from build123d import *

# Parameters (mm, degrees)
SKETCH1_R           = 6.7945
BOSS_EXTRUDE1_DEPTH = 25.4
SKETCH2_W           = 13.589
SKETCH2_H           = 1.500538131
BOSS_EXTRUDE2_DEPTH = 13.97
BOSS_EXTRUDE3_DEPTH = 25.4
CUT_EXTRUDE1_DEPTH  = 27.94


with BuildPart() as part:
    # Sketch1 → Boss-Extrude1 (new body)
    with BuildSketch(Plane.XY):
        Circle(SKETCH1_R)
    extrude(amount=-BOSS_EXTRUDE1_DEPTH)

    # Sketch2 → Boss-Extrude2 (add)
    with BuildSketch(Plane(origin=(0, 0, 0), x_dir=(1, 0, 0), z_dir=(0, 1, 0))):
        with Locations((0, 24.649730935)):
            Rectangle(SKETCH2_W, SKETCH2_H)
    extrude(amount=BOSS_EXTRUDE2_DEPTH)

    # Sketch6 → Boss-Extrude3 (add)
    with BuildSketch(Plane(origin=(0, 13.97, 0), x_dir=(1, 0, 0), z_dir=(0, 1, 0))):
        Polygon((-20.876229987, 25.399999851), (18.493770013, 25.40000027), (18.6055, 0), (-20.876229987, 0), align=None)
    extrude(amount=BOSS_EXTRUDE3_DEPTH)

    # Sketch11 → Cut-Extrude1 (cut)
    with BuildSketch(Plane.XY):
        Polygon((0, 21.022742384), (-12.580876385, 21.022742384), (-12.580876385, 29.426569926), (-6.246648163, 29.426569926), (-6.246648163, 39.37), (0, 39.37), (6.233662889, 39.37), (6.233662889, 29.426569926), (12.693321373, 29.426569926), (12.693321373, 21.022742384), align=None)
    extrude(amount=-CUT_EXTRUDE1_DEPTH, mode=Mode.SUBTRACT)


solid = part.part
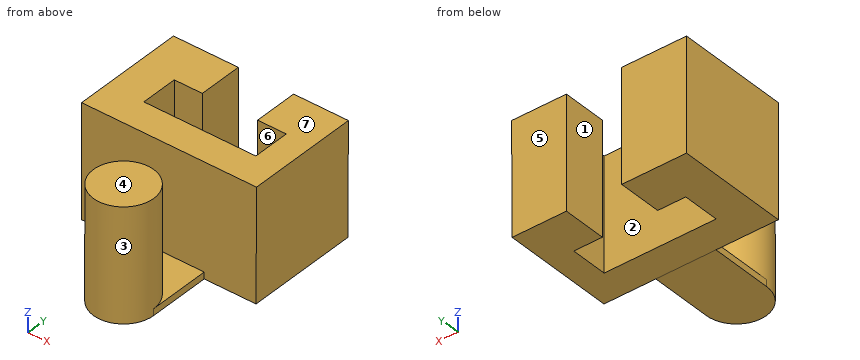
Read the model definition and answer for the solid it produces. Units are mm, in the model's axes. Face numbers are marked on the shaded views. A direction names the side the tool comes from. Give positions to 0.01 mm unless a question says otherwise; leave off trailing zeros. Write each loop counter-clockwise with the first axis right and the second up, starting at its lowest first coordinate (ties: lowest second). Pieces come first, ordered by that corner, then holes. Notation, with made-up numbers: (-25, -2.75) - (20, -2.75) arc R26 cw to (20, 28.25) - close; hole circle Ø1 at (57.25, 74.5). An arc over 180 degrees is marked (long way). Return JSON: item names as keys, results as strings.
Q1. Consider line 1 along Y through (x, z) = (9, -21.5); line 2 along Z through (x, y) = (4.5, 6); line 3 along Y through (x, z) = (-17, -7.25). Determine where each line is inside the solid, lowest interval first. Write a range as [from, to].
Reply:
{"line 1": "[13.97, 21.02], [29.43, 39.37]", "line 2": "[-25.4, -23.9]", "line 3": "[13.97, 39.37]"}
Q2. A cutting plane is placed at B-B, the plane y = 24.5. Determine the outline of the cut face in (x, z).
Reply:
{"outline": "(-20.88, -25.4) - (-12.58, -25.4) - (-12.58, 0) - (-20.88, 0) - close; (12.69, -25.4) - (18.49, -25.4) - (18.61, 0) - (12.69, 0) - close"}
Q3. Given P1, Ø6.5, axis at y = 26, z = -14.5, coming from the +X side; P2, Ø6, axis at x = -7.5, z = -13.5, coming from the -Y side; P3, Ø2, axis at y = -1.5, z = -11.5, coming from the +X side, each flat-ended and moving along its own axis, determine where each tip first touches the part or whether it passes through.
Reply:
{"P1": "x = 18.56", "P2": "y = -5.09", "P3": "x = 6.78"}
Q4. A cutting plane is placed at A-A, the plane x = -7.5. Determine the outline of the cut face in (y, z).
Reply:
{"outline": "(13.97, -25.4) - (21.02, -25.4) - (21.02, 0) - (13.97, 0) - close; (29.43, -25.4) - (39.37, -25.4) - (39.37, 0) - (29.43, 0) - close"}
Q5. A cutting plane is placed at C-C, the plane x = 0. Determine the outline of the cut face in (y, z), and give its area (3 significant figures).
Reply:
{"outline": "(-6.79, -25.4) - (21.02, -25.4) - (21.02, 0) - (13.97, 0) - (13.97, -23.9) - (6.79, -23.9) - (6.79, 0) - (-6.79, 0) - close", "area": "535 mm²"}
Q6. For a pull along Y with two mould halves and no side action, classify the marked faces 5, 6 and 7 as released by +Y, released by -Y, zero draft, split by the parting line, or undercut.
Reply:
{"face 5": "released by +Y", "face 6": "undercut", "face 7": "zero draft"}
Q7. A cutting plane is placed at D-D, the plane z = -17. Determine the outline of the cut face in (x, y).
Reply:
{"outline": "(-20.88, 13.97) - (18.53, 13.97) - (18.53, 39.37) - (6.23, 39.37) - (6.23, 29.43) - (12.69, 29.43) - (12.69, 21.02) - (-12.58, 21.02) - (-12.58, 29.43) - (-6.25, 29.43) - (-6.25, 39.37) - (-20.88, 39.37) - close; circle Ø13.59 at (0, 0)"}
Q8. For the marked faces 1, 2, 3 and 4, determine the directions among +Z, -Z, +X, -X, +Y, -Y from which every point of the face is accessible in a straight line to the end or side of a thin tool.
Reply:
{"face 1": "+Z, -Z, +Y", "face 2": "+Z, -Z", "face 3": "+Z", "face 4": "+Z, +X, -X, +Y, -Y"}
